Geometry check sheet. Reference: the model listing, model coordinates, mm. A direction names the side the tool comes from. Round coordinates to 2 decimals unless told otherwise and drop trailing zeros. Write each loop counter-clockwise with the first axis right and the second up, starting at its lowest first coordinate (ties: lowest second). Pieces come first, ordered by that corner, then holes. Notation, with made-up numbers: (32.25, 27.25) -> (51.25, 27.25) arc R23 cw to (51.25, 43.25) -> close; hole circle Ø8 at (-31.75, 32). An arc over 180 degrees is marked (long way). Use a Markdown table: item, result.
```python
from build123d import *

# Parameters (mm, degrees)
F1_DEPTH = 5.08


# Not quite as in the source:
# - ends of sketch curves that miss each other by under 0.0002 mm in the source are joined


with BuildPart() as f1:
    # F0 (on Front) → F1 (new body)
    with BuildSketch(Plane.XZ):
        with BuildLine():
            ThreePointArc((-12.7, -9.5504), (-12.1920000057, -10.0583238), (-12.6998476, -10.5663999771))
            ThreePointArc((-12.6998476, -10.5663999771), (-12.0825225161, -12.0825225161), (-10.5664000074, -12.6998469825))
            ThreePointArc((-10.5664000074, -12.6998469825), (-10.0583238, -12.1920000057), (-9.5504, -12.7))
            Line((-9.5504, -12.7), (-6.3330836, -12.7))
            ThreePointArc((-6.3330836, -12.7), (-5.8250836, -12.192), (-5.3170836, -12.7))
            Line((-5.3170836, -12.7), (-4.3434, -12.7))
            ThreePointArc((-4.3434, -12.7), (-3.2385, -11.5951), (-4.3434, -10.4902))
            Line((-4.3434, -10.4902), (-6.4747902, -10.4902))
            ThreePointArc((-6.4747902, -10.4902), (-7.413451805, -9.8630063673), (-7.1932106897, -8.7557795103))
            Line((-7.1932106897, -8.7557795103), (-3.8631622, -5.4257448))
            ThreePointArc((-3.8631622, -5.4257448), (-2.8331268978, -4.7374824843), (-1.618107, -4.4958))
            Line((-1.618107, -4.4958), (1.618107, -4.4958))
            ThreePointArc((1.618107, -4.4958), (2.8331268978, -4.7374824843), (3.8631710303, -5.4257359697))
            Line((3.8631710303, -5.4257359697), (7.1932038, -8.7557864))
            ThreePointArc((7.1932038, -8.7557864), (7.413451805, -9.8630063673), (6.4747902, -10.4902))
            Line((6.4747902, -10.4902), (4.3434, -10.4902))
            ThreePointArc((4.3434, -10.4902), (3.2385, -11.5951), (4.3434, -12.7))
            Line((4.3434, -12.7), (5.3170836, -12.7))
            ThreePointArc((5.3170836, -12.7), (5.8250836, -12.192), (6.3330836, -12.7))
            Line((6.3330836, -12.7), (9.5504, -12.7))
            ThreePointArc((9.5504, -12.7), (10.0583238, -12.1920000057), (10.5663999771, -12.6998476))
            ThreePointArc((10.5663999771, -12.6998476), (12.0825225161, -12.0825225161), (12.6998469825, -10.5664000074))
            ThreePointArc((12.6998469825, -10.5664000074), (12.1920000057, -10.0583238), (12.7, -9.5504))
            Line((12.7, -9.5504), (12.7, -6.3330836))
            ThreePointArc((12.7, -6.3330836), (12.192, -5.8250836), (12.7, -5.3170836))
            Line((12.7, -5.3170836), (12.7, -4.3434))
            ThreePointArc((12.7, -4.3434), (11.5951, -3.2385), (10.4902, -4.3434))
            Line((10.4902, -4.3434), (10.4902, -6.4747902))
            ThreePointArc((10.4902, -6.4747902), (9.8630063673, -7.413451805), (8.7557795103, -7.1932106897))
            Line((8.7557795103, -7.1932106897), (5.4257448, -3.8631622))
            ThreePointArc((5.4257448, -3.8631622), (4.7374824843, -2.8331268978), (4.4958, -1.618107))
            Line((4.4958, -1.618107), (4.4958, 1.618107))
            ThreePointArc((4.4958, 1.618107), (4.7374824843, 2.8331268978), (5.4257359697, 3.8631710303))
            Line((5.4257359697, 3.8631710303), (8.7557864, 7.1932038))
            ThreePointArc((8.7557864, 7.1932038), (9.8630063673, 7.413451805), (10.4902, 6.4747902))
            Line((10.4902, 6.4747902), (10.4902, 4.3434))
            ThreePointArc((10.4902, 4.3434), (11.5951, 3.2385), (12.7, 4.3434))
            Line((12.7, 4.3434), (12.7, 5.3170836))
            ThreePointArc((12.7, 5.3170836), (12.192, 5.8250836), (12.7, 6.3330836))
            Line((12.7, 6.3330836), (12.7, 9.5504))
            ThreePointArc((12.7, 9.5504), (12.1920000057, 10.0583238), (12.6998476, 10.5663999771))
            ThreePointArc((12.6998476, 10.5663999771), (12.0825225161, 12.0825225161), (10.5664000074, 12.6998469825))
            ThreePointArc((10.5664000074, 12.6998469825), (10.0583238, 12.1920000057), (9.5504, 12.7))
            Line((9.5504, 12.7), (6.3330836, 12.7))
            ThreePointArc((6.3330836, 12.7), (5.8250836, 12.192), (5.3170836, 12.7))
            Line((5.3170836, 12.7), (4.3434, 12.7))
            ThreePointArc((4.3434, 12.7), (3.2385, 11.5951), (4.3434, 10.4902))
            Line((4.3434, 10.4902), (6.4747902, 10.4902))
            ThreePointArc((6.4747902, 10.4902), (7.413451805, 9.8630063673), (7.1932106897, 8.7557795103))
            Line((7.1932106897, 8.7557795103), (3.8631622, 5.4257448))
            ThreePointArc((3.8631622, 5.4257448), (2.8331268978, 4.7374824843), (1.618107, 4.4958))
            Line((1.618107, 4.4958), (-1.618107, 4.4958))
            ThreePointArc((-1.618107, 4.4958), (-2.8331268978, 4.7374824843), (-3.8631710303, 5.4257359697))
            Line((-3.8631710303, 5.4257359697), (-7.1932038, 8.7557864))
            ThreePointArc((-7.1932038, 8.7557864), (-7.413451805, 9.8630063673), (-6.4747902, 10.4902))
            Line((-6.4747902, 10.4902), (-4.3434, 10.4902))
            ThreePointArc((-4.3434, 10.4902), (-3.2385, 11.5951), (-4.3434, 12.7))
            Line((-4.3434, 12.7), (-5.3170836, 12.7))
            ThreePointArc((-5.3170836, 12.7), (-5.8250836, 12.192), (-6.3330836, 12.7))
            Line((-6.3330836, 12.7), (-9.5504, 12.7))
            ThreePointArc((-9.5504, 12.7), (-10.0583238, 12.1920000057), (-10.5663999771, 12.6998476))
            ThreePointArc((-10.5663999771, 12.6998476), (-12.0825225161, 12.0825225161), (-12.6998469825, 10.5664000074))
            ThreePointArc((-12.6998469825, 10.5664000074), (-12.1920000057, 10.0583238), (-12.7, 9.5504))
            Line((-12.7, 9.5504), (-12.7, 6.3330836))
            ThreePointArc((-12.7, 6.3330836), (-12.192, 5.8250836), (-12.7, 5.3170836))
            Line((-12.7, 5.3170836), (-12.7, 4.3434))
            ThreePointArc((-12.7, 4.3434), (-11.5951, 3.2385), (-10.4902, 4.3434))
            Line((-10.4902, 4.3434), (-10.4902, 6.4747902))
            ThreePointArc((-10.4902, 6.4747902), (-9.8630063673, 7.413451805), (-8.7557795103, 7.1932106897))
            Line((-8.7557795103, 7.1932106897), (-5.4257448, 3.8631622))
            ThreePointArc((-5.4257448, 3.8631622), (-4.7374824843, 2.8331268978), (-4.4958, 1.618107))
            Line((-4.4958, 1.618107), (-4.4958, -1.618107))
            ThreePointArc((-4.4958, -1.618107), (-4.7374824843, -2.8331268978), (-5.4257359697, -3.8631710303))
            Line((-5.4257359697, -3.8631710303), (-8.7557864, -7.1932038))
            ThreePointArc((-8.7557864, -7.1932038), (-9.8630063673, -7.413451805), (-10.4902, -6.4747902))
            Line((-10.4902, -6.4747902), (-10.4902, -4.3434))
            ThreePointArc((-10.4902, -4.3434), (-11.5951, -3.2385), (-12.7, -4.3434))
            Line((-12.7, -4.3434), (-12.7, -5.3170836))
            ThreePointArc((-12.7, -5.3170836), (-12.192, -5.8250836), (-12.7, -6.3330836))
            Line((-12.7, -6.3330836), (-12.7, -9.5504))
        make_face()
        with BuildLine():
            ThreePointArc((-2.6035, 0), (0, 2.6035), (2.6035, 0))
            ThreePointArc((2.6035, 0), (0, -2.6035), (-2.6035, 0))
        make_face(mode=Mode.SUBTRACT)
    extrude(amount=F1_DEPTH)


solid = f1.part
```
(1) Thickness scan on line 1 (X direction, y = -3.9, z = 0); line 2 (Z direction, x = 6.25, y = -4.55); line 3 (Z direction, x = 5.25, y = -0.95). Record the ranges inside material, lowest first.
A:
| item | result |
|---|---|
| line 1 | x = -4.5 to -2.6, 2.6 to 4.5 |
| line 2 | z = -12.42 to -10.49, -7.81 to -4.69, 4.69 to 7.81, 10.49 to 12.42 |
| line 3 | z = -12.7 to -10.49, -6.81 to -3.67, 3.67 to 6.81, 10.49 to 12.7 |
(2) Section check B-B on x = 1. Record the cut outline in (y, z), plus the area to 3 significant figures.
A:
| item | result |
|---|---|
| outline | (-5.08, -4.5) -> (0, -4.5) -> (0, -2.4) -> (-5.08, -2.4) -> close; (-5.08, 2.4) -> (0, 2.4) -> (0, 4.5) -> (-5.08, 4.5) -> close |
| area | 21.3 mm2 |
(3) Gauge pin test, flat ends, axial feed: pin 1 Ø1 at (y, z) = (-2, 0.5) entering from -X; pin 2 Ø1 at (x, y) = (0.5, -3) entering from +Z; pin 3 Ø2.5 at (y, z) = (-2, -0.5) entering from +X. Record the tip position at first contact, or that the pin passes through.
A:
| item | result |
|---|---|
| pin 1 | stops at x = -4.5 |
| pin 2 | stops at z = 4.5 |
| pin 3 | stops at x = 4.5 |
(4) Section check A-A on x = 10. Record the cut outline in (y, z), plus the area to 3 significant figures.
A:
| item | result |
|---|---|
| outline | (-5.08, -12.2) -> (0, -12.2) -> (0, -7.34) -> (-5.08, -7.34) -> close; (-5.08, 7.34) -> (0, 7.34) -> (0, 12.2) -> (-5.08, 12.2) -> close |
| area | 49.3 mm2 |
(5) Release check for a two-part mould opening along Z. For faces 1 (the face through (10.069, -2.504, 12.192)), 2 (the face through (-12.7, -3, 8)), 3 (the face through (-4.744, -2.504, 2.849)) record: +Z half, -Z half, draft (parallel to the pull), parting line (faces both ways), or undercut.
A:
| item | result |
|---|---|
| face 1 | +Z half |
| face 2 | draft |
| face 3 | undercut |
(6) Access from +Z, -Z, +X, -X, +Y, -Y to the whole of each face (thin tool, end or side, straight path). Record for faces 4 (the face through (12.7, -3, -5)), 5 (the face through (10.49, -3, 5)).
A:
| item | result |
|---|---|
| face 4 | +Z, -Z, +X, +Y, -Y |
| face 5 | +Y, -Y |
